Can you work these out from the model? Positions are in its coordinate system, mm. A direction names the side the tool comes from. Round coordinates to 2 decimals unless told otherwise and drop trailing zeros. Loops run counter-clockwise (first coordinate to the right, second up) from the corner with the lowest first, then second, coordinate; pieces in that order, holes last.
(1) Will these pins go through, and if not, where does the flat tip stop? pin 1 Ø2 at (x, y) = (-8, 3.5) entering from +Z; pin 2 Ø3.5 at (x, y) = (-12, 3.5) entering from +Z; pin 3 Ø9 at (x, z) = (21, -13) entering from +Y; pin 4 Ø0.9 at (y, z) = (2, -24.5) entering from -X.
(2) I want a section at D-D on x = 20. Write out the boundary of the cut face in (y, z).
(3) Which directions (+Z, -Z, +X, -X, +Y, -Y) give clear straight access to the entire face, cutting with the end or side of a thin tool? Please do faces 5 (the face through (0, 5, -15)), 6 (the face through (-10, 7, -15)), 7 (the face through (0, 1, -4)).
(4) Thinking about a two-plate mould opening in Z: for faces 1 (the face through (3.01, 1.48, -14.37)), 2 (the face through (-0.6, 1.52, -9.43)), 3 (the face through (26.5, 1.5, -14.2)), 4 (the face through (17, 3, -15)), which applies, released by +Z, released by -Z, zero draft, split by the parting line, or undercut?
(5) I want a section at C-C on x = -8. Write out the boundary of the cut face in (y, z).
(6) I want a section at B-B on z = -19.5. Write out the boundary of the cut face in (x, y), plus the area to 3 significant figures.
(7) I want a section at A-A on x = 3.5. Write out the boundary of the cut face in (y, z), plus the area to 3 significant figures.
(8) If I drill on line 1 along X through (y, z) = (0.8, -15); line 2 along X through (y, z) = (3.5, -11.55); line 3 along Y through (x, z) = (-16, -19.2), over which ranges is the centre line in solid material (lowest first)?
from build123d import *

# Parameters (mm, degrees)
SKETCH1_W             = 30
SKETCH1_H             = 15
BOSS_EXTRUDE1_DEPTH   = 3
SKETCH2_W             = 5
SKETCH2_H             = 7
BOSS_EXTRUDE2_DEPTH   = 20
CUT_EXTRUDE1_DEPTH    = 18
FILLET2_R             = 2
FILLET3_R             = 1
M2X0_4_TAPPED_HOLE1_D = 1.6
M4X0_7_TAPPED_HOLE1_D = 3.3


with BuildPart() as part:
    # Sketch1 → Boss-Extrude1 (new body)
    with BuildSketch(Plane(origin=(0, 0, 0), x_dir=(1, 0, 0), z_dir=(0, 1, 0))):
        with Locations((15, 7.5)):
            Rectangle(SKETCH1_W, SKETCH1_H)
    extrude(amount=BOSS_EXTRUDE1_DEPTH)

    # Sketch2 → Boss-Extrude2 (add)
    with BuildSketch(Plane.ZY):
        with Locations((-12.5, 3.5)):
            Rectangle(SKETCH2_W, SKETCH2_H)
    extrude(amount=BOSS_EXTRUDE2_DEPTH)

    # Sketch3 → Cut-Extrude1 (cut)
    with BuildSketch(Plane.ZY.offset(20)):
        with BuildLine():
            Line((-15, 1), (-15, 6))
            ThreePointArc((-15, 6), (-12.5, 3.5), (-15, 1))
        make_face()
    extrude(amount=-CUT_EXTRUDE1_DEPTH, mode=Mode.SUBTRACT)

    # Mirror1: part across plane


with BuildPart() as part_1:
    add(part.part)
    add(part.part.mirror(Plane(origin=(0, 3, -15), x_dir=(1, 0, 0), z_dir=(0, 0, 1))))

    # Fillet2
    fillet2_edges = [part_1.edges().sort_by_distance(p)[0] for p in [
        (0, 1.5, -10),
        (0, 1.5, -20),
    ]]
    fillet(fillet2_edges, radius=FILLET2_R)

    # Fillet3
    fillet3_edges = [part_1.edges().sort_by_distance(p)[0] for p in [
        (0, 5, -10),
        (-20, 3.5, -10),
        (0, 1.5, -30),
        (30, 1.5, -30),
        (-20, 3.5, -20),
        (0, 5, -20),
        (30, 1.5, 0),
        (0, 1.5, 0),
    ]]
    fillet(fillet3_edges, radius=FILLET3_R)

    # M2x0.4 Tapped Hole1 (through all)
    with Locations(Plane(origin=(3.5, 3, -15), x_dir=(0, 0, 1), z_dir=(0, 1, 0))):
        with Locations((0, 0), (0, 23)):
            Hole(M2X0_4_TAPPED_HOLE1_D / 2)

    # M4x0.7 Tapped Hole1 (through all)
    with Locations(Plane(origin=(-16, 3.5, -10), x_dir=(1, 0, 0), z_dir=(0, 0, 1))):
        with Locations((0, 0), (8, 0)):
            Hole(M4X0_7_TAPPED_HOLE1_D / 2)


solid = part_1.part
Filled sheet:
1. pin 1: passes through
1. pin 2: stops at z = -10
1. pin 3: stops at y = 3
1. pin 4: stops at x = 0
2. outline: (0, -30) - (3, -30) - (3, 0) - (0, 0) - close
3. face 5: +Z, -Z, +X, +Y
3. face 6: +Z, -Z, +X, -X, +Y
3. face 7: +Z, -X, +Y, -Y
4. face 1: undercut
4. face 2: released by +Z
4. face 3: undercut
4. face 4: zero draft
5. outline: (0, -20) - (1.85, -20) - (1.85, -16.88) arc R2.5 cw to (1.85, -13.12) - (1.85, -10) - (0, -10) - close; (5.15, -20) - (7, -20) - (7, -10) - (5.15, -10) - (5.15, -13.12) arc R2.5 cw to (5.15, -16.88) - close
6. outline: (-19.87, 0) - (30, 0) - (30, 3) - (-0.13, 3) - (-0.13, 7) - (-19.87, 7) - close; hole circle Ø3.3 at (-16, 3.5); hole circle Ø3.3 at (-8, 3.5)
6. area: 211 mm2
7. outline: (0, -30) - (3, -30) - (3, -15.8) - (0, -15.8) - close; (0, -14.2) - (3, -14.2) - (3, 0) - (0, 0) - close
7. area: 85.2 mm2
8. line 1: x = -20 to 2.7, 4.3 to 25.7, 27.3 to 30
8. line 2: x = -20 to -17.65, -14.35 to -9.65, -6.35 to 0
8. line 3: y = 0 to 1.85, 5.15 to 7
